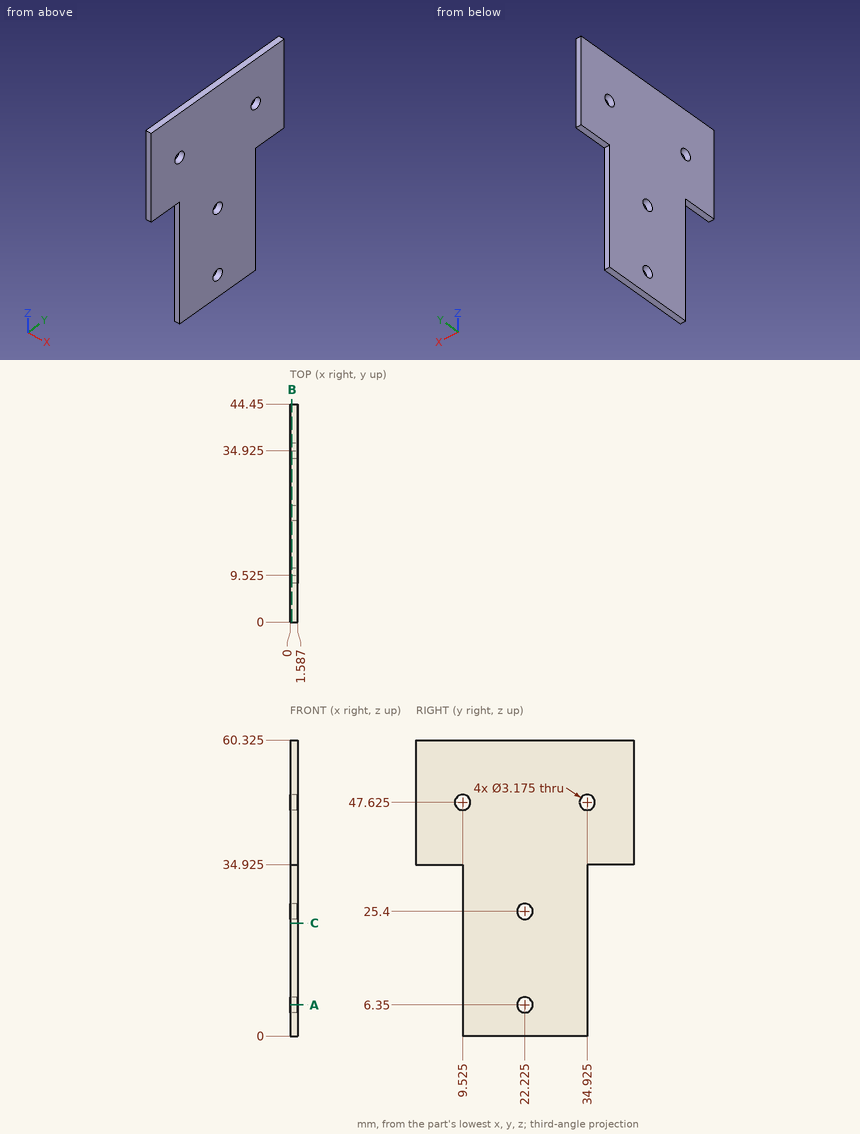
Source: three-view drawing plus pictorial views. Frame: mm from the lowest corner of the part. Give positions to 0.01 mm unless a question says otherwise; leave off trailing zeros. Loops run counter-clockwise (first coordinate to the right, second up) from the corner with the lowest first, then second, coordinate; pieces in that order, holes last. Notation, with made-up numbers: M 58.25,-32.5 L 64.25,-32.5 A32 cw 64.25,-6.5 Z; hole C 57,41.5 d9. An arc over 180 degrees is marked long. Use CSV: the item, a comma, the result in double quotes.
(1) Section A-A, the plane z = 6.35. Return loops of the section in (x, y) (1 decimal).
Outcome:
outline,"M 0,9.5 L 1.6,9.5 L 1.6,20.6 L 0,20.6 Z; M 0,23.8 L 1.6,23.8 L 1.6,34.9 L 0,34.9 Z"
(2) Section C-C, the plane z = 23. Return loops of the section in (x, y) (1 decimal).
Outcome:
outline,"M 0,9.5 L 1.6,9.5 L 1.6,34.9 L 0,34.9 Z"
(3) Section B-B, the plane x = 0.35. Count the separate pieces of the cut face and the enclosed holes in it, plus the area to 3 significant figures.
Outcome:
separate pieces,"1"
enclosed holes,"4"
area,"1,980 mm²"
(4) Pin query (flat end, axial travel): P1, Ø0.5, axis at x = 1, y = 4, coming from the -Z side (1 decimal); P2, Ø1.9, axis at y = 22.225, z = 25.4, coming from the -X side (3 decimals). Return the tip coordinate at first contact, or that it passes through.
Outcome:
P1,"stops at z = 34.9"
P2,"passes through"
(5) Material intervals for L1, parallel to Y at x = 0.9, z = 15 (1 decimal); L2, parallel to Z at x = 0.6, y = 33.5 (1 decimal); L3, parallel to Z at x = 0.9, y = 21 (1 decimal), sorted ascending. Write a range as [from, to].
Outcome:
L1,"y = [9.5, 34.9]"
L2,"z = [0, 46.9], [48.3, 60.3]"
L3,"z = [0, 5.3], [7.4, 24.4], [26.4, 60.3]"
